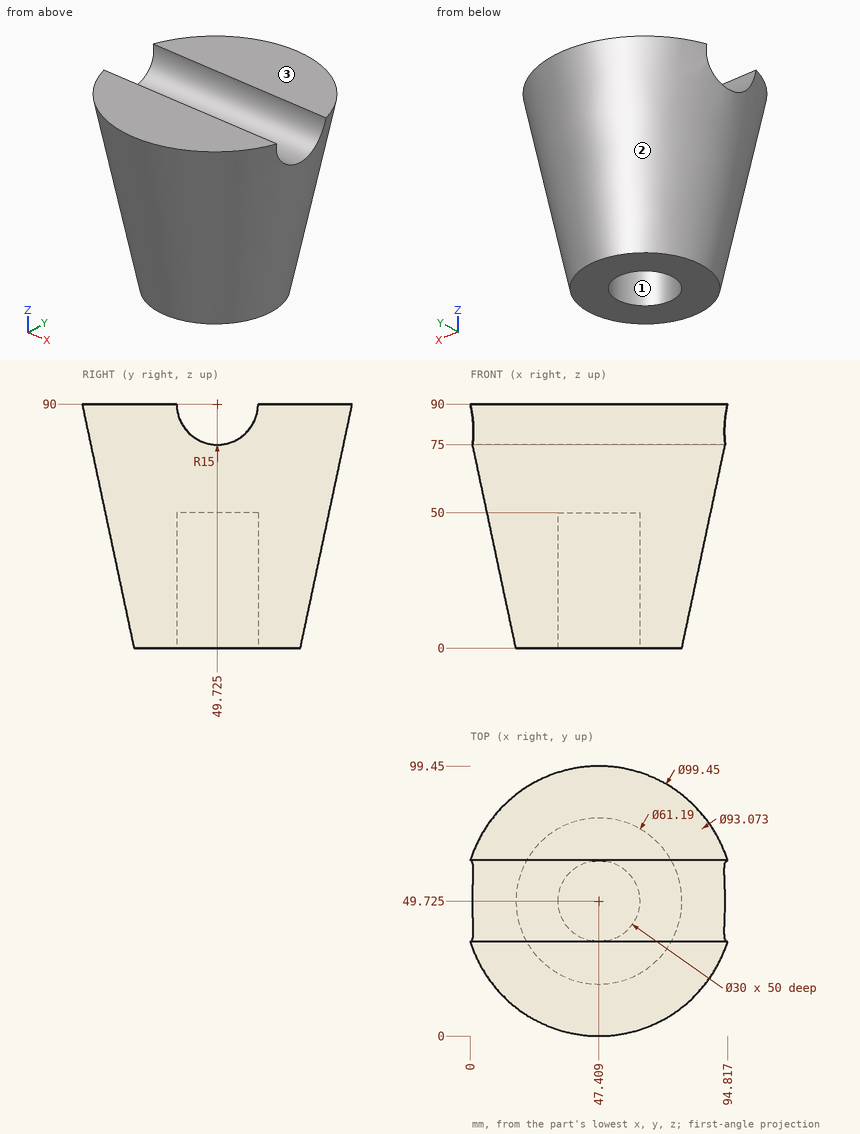
Source: three-view drawing plus pictorial views. Frame: mm from the lowest corner of the part. Round coordinates to 2 decimals unless told otherwise and drop trailing zeros. Use CSV: the item, a comma, the result in double quotes. Start each with the question number.
1) Draft query along Y for the marked faces 1, 2 and 3. Return one class per face: +Y half, -Y half, draft (parallel to the pull), parting line (faces both ways), or undercut.
2) Material intervals for line 1 along X through (y, z) = (50, 29.5) (1 decimal); line 2 along Y through (x, z) = (37, 7.5) (1 decimal); line 3 along Y through (x, z) = (16, 83) (1 decimal), sorted ascending. Write a range as from..to.
3) First-contact query: pin 1 Ø12 at (x, y) = (29, 49.5) entering from +Z; pin 2 Ø2 at (y, z) = (51.5, 41.5) entering from -X (1 decimal); pin 3 Ø6 at (y, z) = (80, 65) entering from -X (1 decimal). Flat tips, straight axial feed; report the tip coordinate or a pass-through.
Returned:
1,face 1,"undercut"
1,face 2,"parting line"
1,face 3,"draft"
2,line 1,"x = 10.5..32.4, 62.4..84.3"
2,line 2,"y = 19.3..38.9, 60.5..80.2"
2,line 3,"y = 13.1..36.5, 63..86.3"
3,pin 1,"stops at z = 76.35"
3,pin 2,"stops at x = 7.8"
3,pin 3,"stops at x = 12.2"
